Autodesk Inventor part; units mm, degrees
ref_plane "IP_screw_XY" through (2.5, 0, 0) normal (1, 0, 0) x (0, 0, -1)
ref_plane "IP_screw_YZ" through (2.5, 0, 0) normal (0, 0, -1) x (0, 1, 0)
ref_plane "IP_screw_ZX" through (2.5, 0, 0) normal (0, 1, 0) x (1, 0, 0)
sketch "Sketch_1" plane through (0, 0, 0) normal (0, 0, 1) x (1, 0, 0)
  line L0 (8.5, 0) -> (0, 0)
  line L1 (0, 0) -> (0, 2.7)
  line L2 (0, 2.7) -> (0.3, 3)
  line L3 (0.3, 3) -> (2.2, 3)
  line L4 (2.2, 3) -> (2.5, 2.7)
  line L5 (2.5, 2.7) -> (2.5, 2.5)
  line L6 (2.5, 2.5) -> (4.8, 2.5)
  line L7 (4.8, 2.5) -> (5, 2.3)
  line L8 (5, 2.3) -> (5, 2)
  line L9 (5, 2) -> (8.0705, 2)
  line L10 (8.0705, 2) -> (8.5, 1.5705)
  line L11 (8.5, 1.5705) -> (8.5, 0)
  line L12 (8.5, 0) -> (0, 0)
revolve "Revolution1" add sketch "Sketch_1" angle 360 about axis through (8.5, 0, 0) along (1, 0, 0)
thread "Thread1"
sketch "Sketch_2" plane through (0, 0, 0) normal (0, 0, 1) x (1, 0, 0)
  line L0 (8.5, 0) -> (0, 0)
  line L1 (0, 0) -> (0, 1.85)
  line L2 (0, 1.85) -> (0.1, 1.75)
  line L3 (0.1, 1.75) -> (4, 1.75)
  line L4 (4, 1.75) -> (4, 1.29)
  line L5 (4, 1.29) -> (4.24, 1.05)
  line L6 (4.24, 1.05) -> (8.26, 1.05)
  line L7 (8.26, 1.05) -> (8.5, 1.29)
  line L8 (8.5, 1.29) -> (8.5, 0)
  line L9 (8.5, 0) -> (0, 0)
revolve "Revolution2" cut sketch "Sketch_2" angle 360 about axis through (8.5, 0, 0) along (1, 0, 0)
sketch "Sketch_3" plane through (8.5, 0, 0) normal (1, 0, 0) x (0, 1, 0)
  line L0 (-1, -0.5774) -> (0, -1.1547)
  line L1 (0, -1.1547) -> (1, -0.5774)
  line L2 (1, -0.5774) -> (1, 0.5774)
  line L3 (1, 0.5774) -> (0, 1.1547)
  line L4 (0, 1.1547) -> (-1, 0.5774)
  line L5 (-1, 0.5774) -> (-1, -0.5774)
extrude "Extrusion1" cut sketch "Sketch_3" against normal blind 4.5
ref_plane "IP_screw_XY" through (2.5, 0, 0) normal (1, 0, 0) x (0, 0, -1)
ref_plane "IP_screw_YZ" through (2.5, 0, 0) normal (0, 0, -1) x (0, 1, 0)
ref_plane "IP_screw_ZX" through (2.5, 0, 0) normal (0, 1, 0) x (1, 0, 0)
properties part number "VPM46-6"
CAD build for the part. Positions are in the model's coordinates, mm. A direction names the side the tool comes from. Coordinates: 2 decimals unless noted, no trailing zeros. Write each loop counter-clockwise with the first axis right and the second up, starting at its lowest first coordinate (ties: lowest second). Pieces come first, ordered by that corner, then holes. Notation, with made-up numbers: M 79.25,-36.75 L 111.25,-36.75 A27 ccw 111.25,-2.75 Z; hole C 41.5,-38 d10. An arc over 180 degrees is marked long. Answer as a JSON object with one key per item and string values. Group by question number.
1) Saw through at C-C (x = 6). Write the cut outline in (y, z), plus the area to 3 significant figures.
2) Saw through at A-A (x = 4.5). Write the cut outline in (y, z).
3) Mould opens along Y. For faces 1 (the face through (0, -1, -2)), 2 (the face through (3.67, -0.54, -2.44)), 3 (the face through (2.077, 1.617, -0.67)) say: +Y half, -Y half, draft (parallel to the pull), parting line (faces both ways), or undercut.
4) Pin check, flat tips, straight feed: pin 1 Ø1 at (y, z) = (0.5, -2) entering from -X; pin 2 Ø1 at (y, z) = (0, -0.5) entering from -X. Stop position of each tip, or through.
5) Saw through at D-D (x = 1.5). Write the cut outline in (y, z).
6) Tool access for faces 4 (the face through (1, -3, 0)), 5 (the face through (7, 0, -2)): list every direction of +Z, -Z, +X, -X, +Y, -Y with a clear straight run to the whole face (end or side of a thin tool).
7) Wall check: line 1 (Z direction, x = 1.35, y = 0); line 2 (Z direction, x = 2.75, y = 0); line 3 (Y direction, x = 1.75, z = 0.3). Give the ranges that are in metal, low to high. Write a range as from..to.
Values follow:
{
 "1": {"outline": "C 0,0 d4; hole M -1,-0.58 L -0.78,-0.71 A1.05 ccw -0.22,-1.03 L 0,-1.15 L 0.22,-1.03 A1.05 ccw 0.78,-0.71 L 1,-0.58 L 1,-0.32 A1.05 ccw 1,0.32 L 1,0.58 L 0.78,0.71 A1.05 ccw 0.22,1.03 L 0,1.15 L -0.22,1.03 A1.05 ccw -0.78,0.71 L -1,0.58 L -1,0.32 A1.05 ccw -1,-0.32 Z", "area": "8.97 mm2"},
 "2": {"outline": "C 0,0 d5; hole M -1,-0.58 L -0.78,-0.71 A1.05 ccw -0.22,-1.03 L 0,-1.15 L 0.22,-1.03 A1.05 ccw 0.78,-0.71 L 1,-0.58 L 1,-0.32 A1.05 ccw 1,0.32 L 1,0.58 L 0.78,0.71 A1.05 ccw 0.22,1.03 L 0,1.15 L -0.22,1.03 A1.05 ccw -0.78,0.71 L -1,0.58 L -1,0.32 A1.05 ccw -1,-0.32 Z"},
 "3": {"face 1": "draft", "face 2": "parting line", "face 3": "undercut"},
 "4": {"pin 1": "stops at x = 0", "pin 2": "passes through"},
 "5": {"outline": "C 0,0 d6; hole C 0,0 d3.5"},
 "6": {"face 4": "+X, -X", "face 5": "+X"},
 "7": {"line 1": "z = -3..-1.75, 1.75..3", "line 2": "z = -2.5..-1.75, 1.75..2.5", "line 3": "y = -2.98..-1.72, 1.72..2.98"}
}
